Source: CAD feature listing. Evaluate the final solid. Frame: model axes, mm. A direction names the side the tool comes from. Give positions to 0.01 mm unless a question says otherwise; leave off trailing zeros. Write each loop counter-clockwise with the first axis right and the second up, starting at its lowest first coordinate (ties: lowest second). Pieces come first, ordered by that corner, then holes. Notation, with made-up numbers: M -27.5,32 L 20.5,32 A9 ccw 20.5,45 Z; hole C 88.5,-11.75 d1. An arc over 180 degrees is marked long. Return JSON: item names as keys, results as strings.
```python
from build123d import *

# Parameters (mm, degrees)
F0_W     = 546.1
F0_H     = 355.6
F1_DEPTH = 19.05
F3_D     = 13.49248
F4_W     = 101.6
F4_H     = 228.6
F5_DEPTH = 19.05
F8_D     = 6.5278
F10_D    = 16.66748


with BuildPart() as f1:
    # F0 (on Top) → F1 (new body)
    with BuildSketch(Plane.XY):
        with Locations((-273.05, 177.8)):
            Rectangle(F0_W, F0_H)
    extrude(amount=F1_DEPTH)

    # F3 (through all)
    with Locations(Plane.XY.offset(19.05)):
        with Locations((-501.65, 304.8), (-44.45, 304.8), (-44.45, 50.8), (-501.65, 50.8)):
            Hole(F3_D / 2)

    # F4 (on face) → F5 (cut)
    with BuildSketch(Plane.XY.offset(19.05)):
        with Locations((-50.8, 177.8)):
            Rectangle(F4_W, F4_H)
    extrude(amount=-F5_DEPTH, mode=Mode.SUBTRACT)

    # F8 (through all)
    with Locations(Plane.XY.offset(19.05)):
        with Locations((-273.05, 177.8)):
            Hole(F8_D / 2)

    # F10 (through all)
    with Locations(Plane(origin=(0, 0, 0), x_dir=(1, 0, 0), z_dir=(0, 0, -1))):
        with Locations((-177.8, -193.675), (-368.3, -193.675), (-368.3, -111.125), (-177.8, -111.125)):
            Hole(F10_D / 2)


solid = f1.part
```
1) Draft query along X for faces 1 (the face through (0, 31, 9)), 2 (the face through (-52, 292.1, 10)), 3 (the face through (-494.91, 51.1, 9.39)). Return one class per face: released by +X, released by -X, zero draft, split by the parting line, or undercut.
Numbers:
{"face 1": "released by +X", "face 2": "zero draft", "face 3": "undercut"}
2) Cut plane B-B, the plane y = 304.8. Return the cut outline in (x, z), then the cut area to 3 significant figures.
Numbers:
{"outline": "M -546.1,0 L -508.4,0 L -508.4,19.05 L -546.1,19.05 Z; M -494.9,0 L -51.2,0 L -51.2,19.05 L -494.9,19.05 Z; M -37.7,0 L 0,0 L 0,19.05 L -37.7,19.05 Z", "area": "9,890 mm²"}
3) Cut plane A-A, the plane x = -177.8. Return the cut outline in (y, z).
Numbers:
{"outline": "M 0,0 L 102.79,0 L 102.79,19.05 L 0,19.05 Z; M 119.46,0 L 185.34,0 L 185.34,19.05 L 119.46,19.05 Z; M 202.01,0 L 355.6,0 L 355.6,19.05 L 202.01,19.05 Z"}
4) Cut plane D-D, the plane z = 8.5. Give the number of separate pieces and of enclosed holes in the cut face, then the cut area to 3 significant figures.
Numbers:
{"separate pieces": "1", "enclosed holes": "9", "area": "169,000 mm²"}
5) Contact query for flat-ended pins moving along their axis: pin 1 Ø15 at (x, y) = (-177.8, 193.675) entering from +Z; pin 2 Ø4 at (x, y) = (-164, 131) entering from -Z; pin 3 Ø5.5 at (y, z) = (138.5, 7.5) entering from +X. Output: stop coordinate, or through.
Numbers:
{"pin 1": "passes through", "pin 2": "stops at z = 0", "pin 3": "stops at x = -101.6"}
6) Line query: line 1 (X direction, y = 192.5, z = 14); line 2 (X direction, y = 105, z = 18.5); line 3 (Y direction, x = -368.3, z = 4.25). Output: solid intervals per line, ascending. Write a range as [from, to].
Numbers:
{"line 1": "x = [-546.1, -376.55], [-360.05, -186.05], [-169.55, -101.6]", "line 2": "x = [-546.1, -373.95], [-362.65, -183.45], [-172.15, -101.6]", "line 3": "y = [0, 102.79], [119.46, 185.34], [202.01, 355.6]"}
7) Set-up query: faces 4 (the face through (-376.25, 191.17, 9.66)), 5 (the face through (-52, 63.5, 10)). Return all of +Z, -Z, +X, -X, +Y, -Y with unobstructed straight access to the full face (end or side cutting, diameter ignored); none if empty.
Numbers:
{"face 4": "+Z, -Z", "face 5": "+Z, -Z, +X"}
8) Cut plane C-C, the plane x = -44.45. Return the cut outline in (y, z), then the cut area to 3 significant figures.
Numbers:
{"outline": "M 0,0 L 44.05,0 L 44.05,19.05 L 0,19.05 Z; M 57.55,0 L 63.5,0 L 63.5,19.05 L 57.55,19.05 Z; M 292.1,0 L 298.05,0 L 298.05,19.05 L 292.1,19.05 Z; M 311.55,0 L 355.6,0 L 355.6,19.05 L 311.55,19.05 Z", "area": "1,910 mm²"}
